Geometry: final body of the model. Coordinates: model frame, mm. A direction names the side the tool comes from. Coordinates: 2 decimals unless noted, no trailing zeros. Order: outer loops, then holes, each group sorted by start corner. A loop starts at its lowest first (then second) coordinate and runs counter-clockwise, first axis right, second up. Notation, with made-up numbers: (-22, 78) - (34, 78) arc R5 ccw to (34, 83) - close; hole circle Ø6 at (27.25, -4). An arc over 180 degrees is marked (long way). Use a Markdown table: item, result. Add a question column.
```python
from build123d import *

# Parameters (mm, degrees)
SKETCH1_W               = 38.1
SKETCH1_H               = 25.4
BOSS_EXTRUDE1_DEPTH     = 5.08
CUT_EXTRUDE1_DEPTH      = 47.071427154
CUT_EXTRUDE1_DEPTH_BACK = 47.071427154
SKETCH2_R               = 0.635
SKETCH3_W               = 5.08
SKETCH3_H               = 3.81
CUT_EXTRUDE2_DEPTH      = 47.071427154
SKETCH4_W               = 2.54
SKETCH4_H               = 12.7
CUT_EXTRUDE3_DEPTH      = 47.071427154
BOSS_EXTRUDE2_DEPTH     = 5.08
SKETCH6_W               = 10.16
SKETCH6_H               = 25.4
CUT_EXTRUDE4_DEPTH      = 60.296897052
SKETCH7_W               = 2.54
SKETCH7_H               = 5.08
CUT_EXTRUDE5_DEPTH      = 60.296897052
FILLET1_R               = 1.27
SKETCH8_W               = 2.54
SKETCH8_H               = 10.16
CUT_EXTRUDE6_DEPTH      = 60.296897052
FILLET2_R               = 1.27


with BuildPart() as part:
    # Sketch1 → Boss-Extrude1 (new body)
    with BuildSketch(Plane.XY):
        with Locations((19.05, 12.7)):
            Rectangle(SKETCH1_W, SKETCH1_H)
    extrude(amount=BOSS_EXTRUDE1_DEPTH)

    # Sketch2 → Cut-Extrude1 (cut, two sides: drawn at the far end of the back side and taken through both)
    with BuildSketch(Plane.XY.offset(5.08).offset(-CUT_EXTRUDE1_DEPTH_BACK)):
        with Locations((17.78, 12.7)):
            Circle(SKETCH2_R)
        with Locations((20.32, 12.7)):
            Circle(SKETCH2_R)
    extrude(amount=CUT_EXTRUDE1_DEPTH + CUT_EXTRUDE1_DEPTH_BACK, mode=Mode.SUBTRACT)

    # Sketch3 → Cut-Extrude2 (cut, through all)
    with BuildSketch(Plane(origin=(0, 0, 0), x_dir=(-1, 0, 0), z_dir=(0, 0, -1))):
        with Locations((-25.4, 23.495)):
            Rectangle(SKETCH3_W, SKETCH3_H)
        with Locations((-12.7, 23.495)):
            Rectangle(SKETCH3_W, SKETCH3_H)
    cut_extrude2 = extrude(amount=-CUT_EXTRUDE2_DEPTH, mode=Mode.SUBTRACT)

    # Mirror1: Cut-Extrude2 across plane
    add(cut_extrude2.mirror(Plane.ZX.offset(12.7)), mode=Mode.SUBTRACT)

    # Sketch4 → Cut-Extrude3 (cut, through all)
    with BuildSketch(Plane.XY.offset(5.08)):
        with Locations((36.83, 6.35)):
            Rectangle(SKETCH4_W, SKETCH4_H)
    extrude(amount=-CUT_EXTRUDE3_DEPTH, mode=Mode.SUBTRACT)

    # Sketch5 → Boss-Extrude2 (add, through all)
    with BuildSketch(Plane.XY.offset(5.08)):
        Polygon((38.1, 20.32), (53.34, 20.32), (53.34, 0), (40.64, 0), (40.64, 12.7), (38.1, 12.7), align=None)
    extrude(amount=-BOSS_EXTRUDE2_DEPTH)

    # Sketch6 → Cut-Extrude4 (cut, through all)
    with BuildSketch(Plane.XY.offset(5.08)):
        with Locations((5.08, 12.7)):
            Rectangle(SKETCH6_W, SKETCH6_H)
    extrude(amount=-CUT_EXTRUDE4_DEPTH, mode=Mode.SUBTRACT)

    # Sketch7 → Cut-Extrude5 (cut, through all)
    with BuildSketch(Plane.XY.offset(5.08)):
        with Locations((36.83, 22.86)):
            Rectangle(SKETCH7_W, SKETCH7_H)
    extrude(amount=-CUT_EXTRUDE5_DEPTH, mode=Mode.SUBTRACT)

    # Fillet1
    fillet1_edges = [part.edges().sort_by_distance(p)[0] for p in [
        (35.56, 25.4, 2.54),
        (27.94, 21.59, 2.54),
        (27.94, 25.4, 2.54),
        (22.86, 25.4, 2.54),
        (22.86, 21.59, 2.54),
        (15.24, 21.59, 2.54),
        (15.24, 25.4, 2.54),
        (10.16, 21.59, 2.54),
        (27.94, 0, 2.54),
        (27.94, 3.81, 2.54),
        (22.86, 3.81, 2.54),
        (22.86, 0, 2.54),
        (15.24, 0, 2.54),
        (15.24, 3.81, 2.54),
        (10.16, 3.81, 2.54),
    ]]
    fillet(fillet1_edges, radius=FILLET1_R)

    # Sketch8 → Cut-Extrude6 (cut, through all)
    with BuildSketch(Plane.XY.offset(5.08)):
        with Locations((34.29, 5.08)):
            Rectangle(SKETCH8_W, SKETCH8_H)
    extrude(amount=-CUT_EXTRUDE6_DEPTH, mode=Mode.SUBTRACT)

    # Fillet2
    fillet2_edges = [part.edges().sort_by_distance(p)[0] for p in [
        (53.34, 20.32, 2.54),
        (53.34, 0, 2.54),
        (40.64, 0, 2.54),
    ]]
    fillet(fillet2_edges, radius=FILLET2_R)


solid = part.part
```
1) First-contact query: pin 1 (0.8 mm diameter, centred on x = 34, z = 3.5, fed in from -Y); pin 2 (0.6 mm diameter, centred on y = 23.5, z = 1.5, fed in from -X); pin 3 (2 mm diameter, centred on x = 49, z = 1.5, fed in from +Y). Flat tips, straight axial feed; report the tip coordinate or a pass-through.
2) Section query A-A (y = 9). Return the cut outline in (x, z).
3) Line query: line 1 (Y direction, x = 20.32, z = 1.85) (3 decimals); line 2 (X direction, y = 8.5, z = 3.7); line 3 (X direction, y = 23, z = 2.75). Output: solid intervals per line, ascending. Write a range as from..to.
4) Section query C-C (y = 3). Return the cut outline in (x, z).
5) Section query D-D (x = 36). Return the cut outline in (y, z), and give its area (3 significant figures).
6) Draft query along X for faces 1 (the cylindrical face through (52.958, 0.362, 2.504)), 2 (the flat face through (32, 25.4, 3)), 3 (the cylindrical face through (41.002, 0.382, 2.504)). Return one class per face: released by +X, released by -X, zero draft, split by the parting line, or undercut.
7) Section query B-B (x = 20.32). Return the cut outline in (y, z) (3 decimals).
8) Access query for faces 4 (the flat face through (15.24, 23.5, 2.5)), 5 (the cylindrical face through (27.558, 3.448, 2.576)), 6 (the flat face through (13, 3.81, 3)). Directions: +Z, -Z, +X, -X, +Y, -Y. A direction counts if a zero-diameter tool reaches every point of the face in a straight line with its end or side. Return the directions, or none.
From the geometry:
| question | item | result |
|---|---|---|
| 1 | pin 1 | stops at y = 10.16 |
| 1 | pin 2 | stops at x = 15.24 |
| 1 | pin 3 | stops at y = 20.32 |
| 2 | outline | (10.16, 0) - (33.02, 0) - (33.02, 5.08) - (10.16, 5.08) - close; (40.64, 0) - (53.34, 0) - (53.34, 5.08) - (40.64, 5.08) - close |
| 3 | line 1 | y = 0..12.065, 13.335..25.4 |
| 3 | line 2 | x = 10.16..33.02, 40.64..53.34 |
| 3 | line 3 | x = 15.24..22.86, 27.94..35.56 |
| 4 | outline | (15.15, 0) - (22.95, 0) - (22.95, 5.08) - (15.15, 5.08) - close; (27.85, 0) - (33.02, 0) - (33.02, 5.08) - (27.85, 5.08) - close; (40.64, 0) - (53.34, 0) - (53.34, 5.08) - (40.64, 5.08) - close |
| 5 | outline | (12.7, 0) - (20.32, 0) - (20.32, 5.08) - (12.7, 5.08) - close |
| 5 | area | 38.7 mm^2 |
| 6 | face 1 | released by +X |
| 6 | face 2 | zero draft |
| 6 | face 3 | undercut |
| 7 | outline | (0, 0) - (12.065, 0) - (12.065, 5.08) - (0, 5.08) - close; (13.335, 0) - (25.4, 0) - (25.4, 5.08) - (13.335, 5.08) - close |
| 8 | face 4 | +Z, -Z, -X, +Y |
| 8 | face 5 | +Z, -Z, -Y |
| 8 | face 6 | +Z, -Z, -X, -Y |
